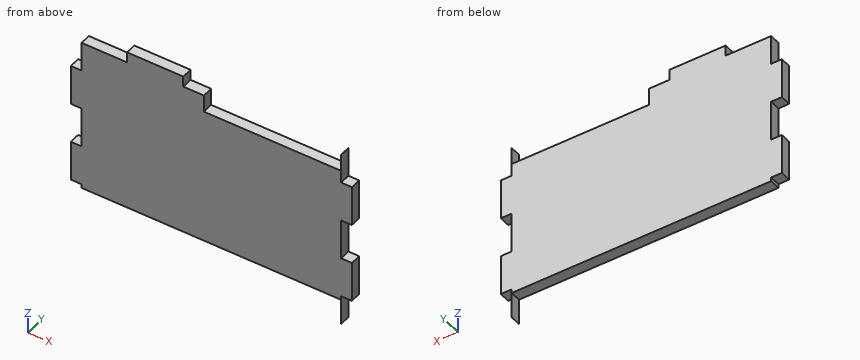
from build123d import *

# Parameters (mm, degrees)
SKETCH1_W           = 83.185
SKETCH1_H           = 59.69
BOSS_EXTRUDE1_DEPTH = 3.175
SKETCH2_W           = 16.637
SKETCH2_H           = 3.175
CUT_EXTRUDE1_DEPTH  = 3.175
LPATTERN1_COUNT     = 3
LPATTERN1_PITCH     = 33.274
SKETCH3_W           = 3.175
SKETCH3_H           = 11.938
CUT_EXTRUDE2_DEPTH  = 3.175
LPATTERN4_COUNT     = 3
LPATTERN4_PITCH     = 23.876
SKETCH5_W           = 76.801567088
SKETCH5_H           = 11.204108434
SKETCH5_W_2         = 40.606567088
SKETCH5_H_2         = 13.017856784
CUT_EXTRUDE4_DEPTH  = 3.175


with BuildPart() as part:
    # Sketch1 → Boss-Extrude1 (new body)
    with BuildSketch(Plane(origin=(0, 0, 0), x_dir=(1, 0, 0), z_dir=(0, 1, 0))):
        Rectangle(SKETCH1_W, SKETCH1_H)
    extrude(amount=BOSS_EXTRUDE1_DEPTH)

    # Sketch2 → Cut-Extrude1 (cut)
    with BuildSketch(Plane(origin=(0, 3.175, 0), x_dir=(1, 0, 0), z_dir=(0, 1, 0))):
        with Locations((-33.274, 28.2575)):
            Rectangle(SKETCH2_W, SKETCH2_H)
        with Locations((-33.274, -28.2575)):
            Rectangle(SKETCH2_W, SKETCH2_H)
    cut_extrude1 = extrude(amount=-CUT_EXTRUDE1_DEPTH, mode=Mode.SUBTRACT)

    # LPattern1: Cut-Extrude1 ×3
    with Locations(*[(i * LPATTERN1_PITCH, 0, 0) for i in range(1, LPATTERN1_COUNT)]):
        add(cut_extrude1, mode=Mode.SUBTRACT)

    # Sketch3 → Cut-Extrude2 (cut)
    with BuildSketch(Plane(origin=(0, 3.175, 0), x_dir=(1, 0, 0), z_dir=(0, 1, 0))):
        with Locations((-40.005, 23.876)):
            Rectangle(SKETCH3_W, SKETCH3_H)
        with Locations((40.005, 23.876)):
            Rectangle(SKETCH3_W, SKETCH3_H)
    cut_extrude2 = extrude(amount=-CUT_EXTRUDE2_DEPTH, mode=Mode.SUBTRACT)

    # LPattern4: Cut-Extrude2 ×3
    with Locations(*[(0, 0, i * LPATTERN4_PITCH) for i in range(1, LPATTERN4_COUNT)]):
        add(cut_extrude2, mode=Mode.SUBTRACT)

    # Sketch5 → Cut-Extrude4 (cut)
    with BuildSketch(Plane(origin=(0, 3.175, 0), x_dir=(1, 0, 0), z_dir=(0, 1, 0))):
        with Locations((-0.016716456, 24.652054217)):
            Rectangle(SKETCH5_W, SKETCH5_H)
        with Locations((18.080783544, -28.098928392)):
            Rectangle(SKETCH5_W_2, SKETCH5_H_2)
    extrude(amount=-CUT_EXTRUDE4_DEPTH, mode=Mode.SUBTRACT)


solid = part.part
The model under review builds one solid part; all positions refer to its coordinate system, in mm. Give positions to 0.01 mm unless a question says otherwise; leave off trailing zeros. Loops run counter-clockwise (first coordinate to the right, second up) from the corner with the lowest first, then second, coordinate; pieces in that order, holes last. Notation, with made-up numbers: (45.25, 7.5) -> (62.25, 7.5) arc R33 ccw to (62.25, 43.5) -> close; hole circle Ø2 at (4.25, 72.5). An arc over 180 degrees is marked (long way). Answer as a JSON object with one key per item and string values. Group by question number.
Q1. Take a section at D-D (z = 1). Write out the cut boundary in (x, y) (1 decimal), plus the area to 3 significant figures.
Q2. Insertion check: pin 1 (1.6 mm diameter, centred on x = -39.5, y = 1, fed in from +Z); pin 2 (1.6 mm diameter, centred on x = -35, y = 1.5, fed in from +Z); pin 3 (0.6 mm diameter, centred on y = 1.5, z = -18.5, fed in from -X); pin 4 (4 mm diameter, centred on x = 27, z = 19.5, fed in from -Y). Each pin has a flat end and moves straight along its axis. Give the tip position at first contact, or say it passes through.
Q3. Take a section at C-C (x = -26). Write out the cut boundary in (y, z) (3 decimals).
Q4. Wall thickness on line 1 along Z through (x, y) = (9, 1.95); line 2 along Z through (x, y) = (-22.5, 1.1) (3 decimals); line 3 along X through (y, z) = (1.7, -4.5): over which ranges is each line inside the solid? List them lowest first.
Answer below:
{
 "1": {"outline": "(-38.4, 0) -> (38.4, 0) -> (38.4, 3.2) -> (-38.4, 3.2) -> close", "area": "244 mm2"},
 "2": {"pin 1": "stops at z = 17.91", "pin 2": "stops at z = 26.67", "pin 3": "stops at x = -38.42", "pin 4": "stops at y = 0"},
 "3": {"outline": "(0, -19.05) -> (3.175, -19.05) -> (3.175, 26.67) -> (0, 26.67) -> close"},
 "4": {"line 1": "z = -19.05 to 21.59", "line 2": "z = -19.05 to 29.845", "line 3": "x = -38.42 to 38.42"}
}
